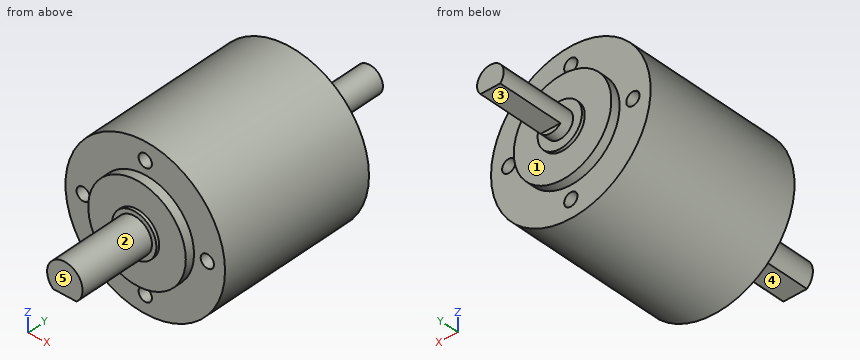
```python
from build123d import *

# Parameters (mm, degrees)
SKETCH1_R           = 18
BOSS_EXTRUDE1_DEPTH = 17.9451
BOSS_EXTRUDE2_START = -17.9451
SKETCH2_R           = 11
BOSS_EXTRUDE2_DEPTH = 20.0025
SKETCH3_R           = 3
BOSS_EXTRUDE4_DEPTH = 18
CUT_EXTRUDE1_DEPTH  = 15
SKETCH5_R           = 1.5
CUT_EXTRUDE2_DEPTH  = 4
SKETCH6_R           = 4
BOSS_EXTRUDE5_DEPTH = 18
CUT_EXTRUDE3_DEPTH  = 15
SKETCH9_R           = 5
BOSS_EXTRUDE6_DEPTH = 20.701


with BuildPart() as part:
    # Sketch1 → Boss-Extrude1 (new body, symmetric)
    with BuildSketch(Plane(origin=(0, 0, 0), x_dir=(1, 0, 0), z_dir=(0, 1, 0))):
        Circle(SKETCH1_R)
    extrude(amount=BOSS_EXTRUDE1_DEPTH, both=True)

    # Sketch2 → Boss-Extrude2 (add, symmetric)
    with BuildSketch(Plane(origin=(0, 17.9451, 0), x_dir=(1, 0, 0), z_dir=(0, 1, 0)).offset(BOSS_EXTRUDE2_START)):
        Circle(SKETCH2_R)
    extrude(amount=BOSS_EXTRUDE2_DEPTH, both=True)

    # Sketch3 → Boss-Extrude4 (add)
    with BuildSketch(Plane(origin=(0, 20.0025, 0), x_dir=(1, 0, 0), z_dir=(0, 1, 0))):
        Circle(SKETCH3_R)
    extrude(amount=BOSS_EXTRUDE4_DEPTH)

    # Sketch4 → Cut-Extrude1 (cut)
    with BuildSketch(Plane(origin=(0, 38.0025, 0), x_dir=(1, 0, 0), z_dir=(0, 1, 0))):
        with BuildLine():
            Line((-2.236067977, 2), (2.236067977, 2))
            ThreePointArc((2.236067977, 2), (0, 3), (-2.236067977, 2))
        make_face()
    cut_extrude1 = extrude(amount=-CUT_EXTRUDE1_DEPTH, mode=Mode.SUBTRACT)

    # Sketch5 → Cut-Extrude2 (cut)
    with BuildSketch(Plane(origin=(0, 17.9451, 0), x_dir=(1, 0, 0), z_dir=(0, 1, 0))):
        with Locations((0, 14)):
            Circle(SKETCH5_R)
        with Locations((-14, 0)):
            Circle(SKETCH5_R)
        with Locations((0, -14)):
            Circle(SKETCH5_R)
        with Locations((14, 0)):
            Circle(SKETCH5_R)
    cut_extrude2 = extrude(amount=-CUT_EXTRUDE2_DEPTH, mode=Mode.SUBTRACT)

    # Mirror1: Cut-Extrude1, Cut-Extrude2 across plane
    add(cut_extrude1.mirror(Plane.ZX), mode=Mode.SUBTRACT)
    add(cut_extrude2.mirror(Plane.ZX), mode=Mode.SUBTRACT)

    # Sketch6 → Boss-Extrude5 (add)
    with BuildSketch(Plane.XZ.offset(20.0025)):
        Circle(SKETCH6_R)
    extrude(amount=BOSS_EXTRUDE5_DEPTH)

    # Sketch7 → Cut-Extrude3 (cut)
    with BuildSketch(Plane.XZ.offset(38.0025)):
        with BuildLine():
            Line((-2.645751311, -3), (2.645751311, -3))
            ThreePointArc((2.645751311, -3), (0, -4), (-2.645751311, -3))
        make_face()
    extrude(amount=-CUT_EXTRUDE3_DEPTH, mode=Mode.SUBTRACT)

    # Sketch9 → Boss-Extrude6 (add, symmetric)
    with BuildSketch(Plane(origin=(0, 0, 0), x_dir=(1, 0, 0), z_dir=(0, 1, 0))):
        Circle(SKETCH9_R)
    extrude(amount=BOSS_EXTRUDE6_DEPTH, both=True)


solid = part.part
```
Geometry: final body of the model. Coordinates: model frame, mm. Face numbers are marked on the shaded views. A direction names the side the tool comes from. Round coordinates to 2 decimals unless told otherwise and drop trailing zeros. Loops run counter-clockwise (first coordinate to the right, second up) from the corner with the lowest first, then second, coordinate; pieces in that order, holes last. Notation, with made-up numbers: (-22, 83) -> (25, 83) arc R15 ccw to (25, 92) -> close; hole circle Ø9 at (78, -32.5). An arc over 180 degrees is marked (long way). Use one line per item in the form item = value. Start each with the question number.
1) Section C-C on x = 10. Output: boundary loops of the cut face in (y, z).
2) Section A-A on y = -15.5. Output: boundary loops of the cut face in (x, z).
3) Section B-B on z = -14. Output: boundary loops of the cut face in (x, y), then the cut area to 3 significant figures.
4) Line query: L1, parallel to Z at x = 0, y = -16; L2, parallel to Y at x = 12.5, z = -7. Output: solid intervals per line, ascending.
5) First-contact query: P1, Ø2.5, axis at x = -14, z = 0, coming from the +Y side; P2, Ø2.5, axis at x = 0, z = 14, coming from the -Y side; P3, Ø5, axis at y = -1, z = -9.5, coming from the -X side. Flat tips, straight axial feed; report the tip coordinate or a pass-through.
6) Access query for the marked faces 1, 2, 3, 4 and 5. Directions: +Z, -Z, +X, -X, +Y, -Y. A direction counts if a zero-diameter tool reaches every point of the face in a straight line with its end or side. Return the directions, or none.
7) Section D-D on y = 32. Output: boundary loops of the cut face in (x, z), then the cut area to 3 significant figures.
Response:
q1.outline = (-20, -4.58) -> (-17.95, -4.58) -> (-17.95, -14.97) -> (17.95, -14.97) -> (17.95, -4.58) -> (20, -4.58) -> (20, 4.58) -> (17.95, 4.58) -> (17.95, 14.97) -> (-17.95, 14.97) -> (-17.95, 4.58) -> (-20, 4.58) -> close
q2.outline = circle Ø36 at (0, 0); hole circle Ø3 at (-14, 0); hole circle Ø3 at (0, -14); hole circle Ø3 at (0, 14); hole circle Ø3 at (14, 0)
q3.outline = (-11.31, -17.95) -> (-1.5, -17.95) -> (-1.5, -13.95) -> (1.5, -13.95) -> (1.5, -17.95) -> (11.31, -17.95) -> (11.31, 17.95) -> (1.5, 17.95) -> (1.5, 13.95) -> (-1.5, 13.95) -> (-1.5, 17.95) -> (-11.31, 17.95) -> close
q3.area = 788 mm^2
q4.L1 = -18 to -15.5, -12.5 to 12.5, 15.5 to 18
q4.L2 = -17.95 to 17.95
q5.P1 = 13.95
q5.P2 = -13.95
q5.P3 = -16.58
q6.face_1 = +Y
q6.face_2 = -Y
q6.face_3 = -Z, +X, -X, +Y
q6.face_4 = -Z, +X, -X, -Y
q6.face_5 = +Z, -Z, +X, -X, -Y
q7.outline = (-2.24, -2) -> (2.24, -2) arc R3 ccw (long way) to start
q7.area = 25.2 mm^2
